Geometry: final body of the model. Coordinates: model frame, mm. A direction names the side the tool comes from. Round coordinates to 2 decimals unless told otherwise and drop trailing zeros. Loops run counter-clockwise (first coordinate to the right, second up) from the corner with the lowest first, then second, coordinate; pieces in that order, holes last. Notation, with made-up numbers: (31, -29) -> (58, -29) arc R11 cw to (58, -23) -> close; hole circle Ø8 at (18, 62.25). An arc over 180 degrees is marked (long way). Answer in a Markdown table with one row per item.
```python
from build123d import *

# Parameters (mm, degrees)
SKETCH1_R           = 5
SKETCH1_R_2         = 4
BOSS_EXTRUDE1_DEPTH = 10.5
BOSS_EXTRUDE2_START = -2
SKETCH2_R           = 11
SKETCH2_R_2         = 4.5
BOSS_EXTRUDE2_DEPTH = 3.5
SKETCH3_R           = 1.5
CUT_EXTRUDE1_DEPTH  = 18.727097901


with BuildPart() as part:
    # Sketch1 → Boss-Extrude1 (new body)
    with BuildSketch(Plane(origin=(0, 0, 0), x_dir=(1, 0, 0), z_dir=(0, 1, 0))):
        with Locations(Location((0, 0, 0), (0, 0, 90))):
            Circle(SKETCH1_R)
        with Locations(Location((0, 0, 0), (0, 0, 90))):
            Circle(SKETCH1_R_2, mode=Mode.SUBTRACT)
    extrude(amount=BOSS_EXTRUDE1_DEPTH)

    # Sketch2 → Boss-Extrude2 (add)
    with BuildSketch(Plane(origin=(0, 10.5, 0), x_dir=(1, 0, 0), z_dir=(0, 1, 0)).offset(BOSS_EXTRUDE2_START)):
        with Locations(Location((0, 0, 0), (0, 0, 270))):
            Circle(SKETCH2_R)
        Circle(SKETCH2_R_2, mode=Mode.SUBTRACT)
    extrude(amount=-BOSS_EXTRUDE2_DEPTH)

    # Sketch3 → Cut-Extrude1 (cut, through all)
    with BuildSketch(Plane(origin=(0, 8.5, 0), x_dir=(1, 0, 0), z_dir=(0, 1, 0))):
        with Locations(Location((-5.75, 5.75, 0), (0, 0, 270))):
            Circle(SKETCH3_R)
        with Locations(Location((5.75, 5.75, 0), (0, 0, 270))):
            Circle(SKETCH3_R)
        with Locations(Location((5.75, -5.75, 0), (0, 0, 270))):
            Circle(SKETCH3_R)
        with Locations(Location((-5.75, -5.75, 0), (0, 0, 270))):
            Circle(SKETCH3_R)
    extrude(amount=-CUT_EXTRUDE1_DEPTH, mode=Mode.SUBTRACT)


solid = part.part
```
Item 1: First-contact query: P1, Ø5, axis at x = -5.75, z = -5.75, coming from the -Y side; P2, Ø1, axis at x = 7, y = 8, coming from the +Z side; P3, Ø2, axis at y = 6.5, z = 3, coming from the +X side. Flat tips, straight axial feed; report the tip coordinate or a pass-through.
Ans:
| item | result |
|---|---|
| P1 | y = 5 |
| P2 | z = 8.87 |
| P3 | x = 10.82 |
Item 2: Mould query, pull axis Z, two halves, no side actions, for faces 3 (the cylindrical face through (-5.68, 6.77, 4.25)), 4 (the flat face through (-2, 5, 5)), 5 (the cylindrical face through (4.88, 2.46, 1.08)). Classes: released by +Z, released by -Z, zero draft, split by the parting line, or undercut.
Ans:
| item | result |
|---|---|
| face 3 | undercut |
| face 4 | zero draft |
| face 5 | split by the parting line |
Item 3: Section query D-D, the plane x = -1. Output: boundary loops of the cut face in (y, z), and give its area (3 significant figures).
Ans:
| item | result |
|---|---|
| outline | (0, -4.9) -> (5, -4.9) -> (5, -10.95) -> (8.5, -10.95) -> (8.5, -4.9) -> (10.5, -4.9) -> (10.5, -3.87) -> (0, -3.87) -> close; (0, 3.87) -> (10.5, 3.87) -> (10.5, 4.9) -> (8.5, 4.9) -> (8.5, 10.95) -> (5, 10.95) -> (5, 4.9) -> (0, 4.9) -> close |
| area | 63.9 mm2 |
Item 4: Ray query, L1, parallel to Z at x = -5.5, y = 8; L2, parallel to X at y = 7.55, z = 5.75; L3, parallel to X at y = 5.25, z = -6.25. Return the intervals inside material, ascending.
Ans:
| item | result |
|---|---|
| L1 | -9.53 to -7.23, -4.27 to 4.27, 7.23 to 9.53 |
| L2 | -9.38 to -7.25, -4.25 to 4.25, 7.25 to 9.38 |
| L3 | -9.05 to -7.16, -4.34 to 4.34, 7.16 to 9.05 |
Item 5: Section query A-A, the plane z = 0. Output: boundary loops of the cut face in (x, y).
Ans:
| item | result |
|---|---|
| outline | (-11, 5) -> (-5, 5) -> (-5, 0) -> (-4, 0) -> (-4, 10.5) -> (-5, 10.5) -> (-5, 8.5) -> (-11, 8.5) -> close; (4, 0) -> (5, 0) -> (5, 5) -> (11, 5) -> (11, 8.5) -> (5, 8.5) -> (5, 10.5) -> (4, 10.5) -> close |
Item 6: Section query B-B, the plane x = -5.75. Output: boundary loops of the cut face in (y, z).
Ans:
| item | result |
|---|---|
| outline | (5, -9.38) -> (8.5, -9.38) -> (8.5, -7.25) -> (5, -7.25) -> close; (5, -4.25) -> (8.5, -4.25) -> (8.5, 4.25) -> (5, 4.25) -> close; (5, 7.25) -> (8.5, 7.25) -> (8.5, 9.38) -> (5, 9.38) -> close |
Item 7: Section query C-C, the plane y = 7.5. Output: boundary loops of the cut face in (x, z).
Ans:
| item | result |
|---|---|
| outline | circle Ø22 at (0, 0); hole circle Ø3 at (-5.75, -5.75); hole circle Ø3 at (-5.75, 5.75); hole circle Ø8 at (0, 0); hole circle Ø3 at (5.75, -5.75); hole circle Ø3 at (5.75, 5.75) |
Item 8: Set-up query: faces 1 (the flat face through (-2, 8.5, 5)), 2 (the cylindrical face through (5.82, 6.77, -7.25)). Return all of +Z, -Z, +X, -X, +Y, -Y with unobstructed straight access to the full face (end or side cutting, diameter ignored); none if empty.
Ans:
| item | result |
|---|---|
| face 1 | +Y |
| face 2 | +Y, -Y |
